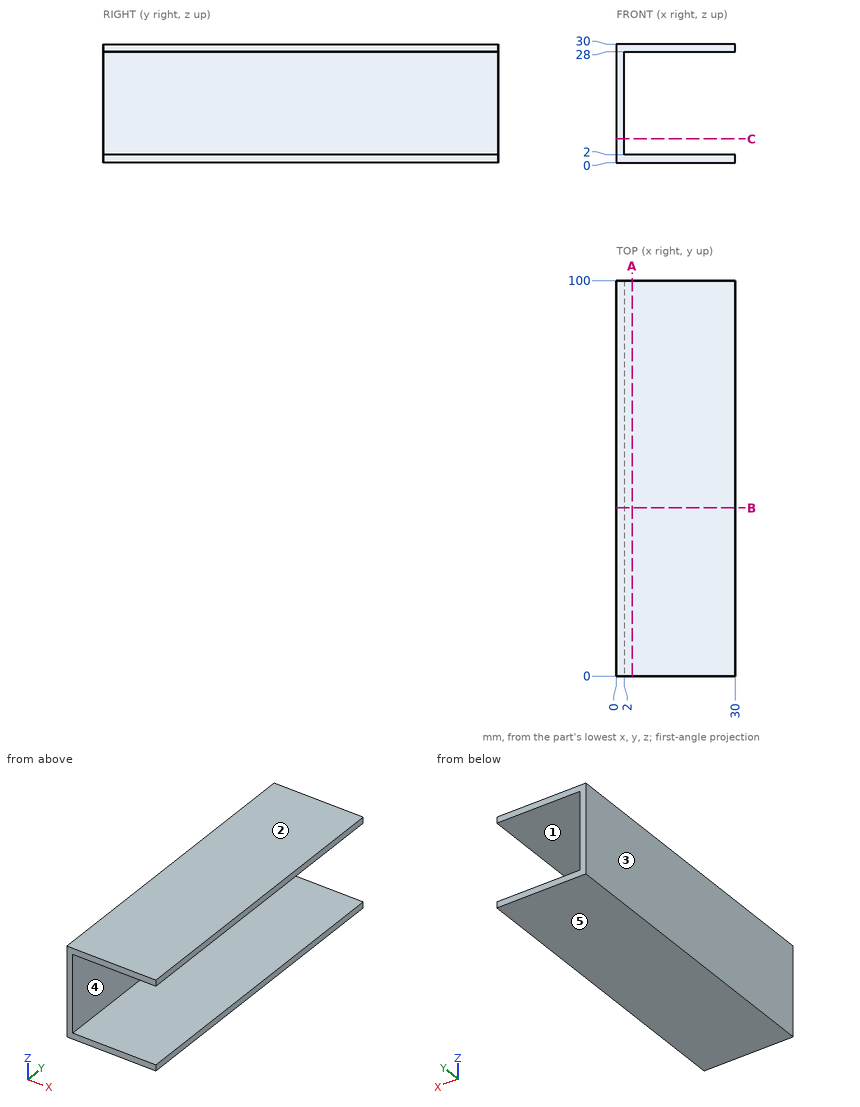
Geometry check sheet. Reference: drawing and pictorial views, mm from the part's lowest x, y, z. A direction names the side the tool comes from. Round coordinates to 2 decimals unless told otherwise and drop trailing zeros. Loops run counter-clockwise (first coordinate to the right, second up) from the corner with the lowest first, then second, coordinate; pieces in that order, holes last. Notation, with made-up numbers: (68.5, 1) - (77.5, 1) arc R23 ccw to (77.5, 28) - close; hole circle Ø8 at (-33, -22.5). An arc over 180 degrees is marked (long way). Answer in a Markdown table with one row per item. Add a question column.
Q1. Section check A-A on x = 4. Enter the section's corners in (y, z), plus the area to 3 significant figures.
Q2. Material ranges on line 1 (Z direction, x = 13.5, y = 51); line 2 (X direction, y = 25, z = 25.5), recorded low to high.
Q3. Section check C-C on z = 6. Enter the section's corners in (x, y).
Q4. Section check B-B on y = 42.5. Enter the section's corners in (x, z).
Q5. Release check for a two-part mould opening along Z. For the marked faces 3, 4 and 5 record: pulls with the +Z half, pulls with the -Z half, needs draft (parallel to the pull), parting line crosses it, or undercut.
Q6. Gauge pin test, flat end, axial feed: pin 1 (8.5 mm diameter, centred on x = 22, y = 26, fed in from -Z). Record the tip position at first contact, or that the pin passes through.
Q7. Tool access check on the marked faces 1 and 2. Record the directions out of +Z, -Z, +X, -X, +Y, -Y that give a thin tool (end or side, any length) a straight path to the whole face; none if there is none.
Found:
| question | item | result |
|---|---|---|
| 1 | outline | (0, 0) - (100, 0) - (100, 2) - (0, 2) - close; (0, 28) - (100, 28) - (100, 30) - (0, 30) - close |
| 1 | area | 400 mm² |
| 2 | line 1 | z = 0 to 2, 28 to 30 |
| 2 | line 2 | x = 0 to 2 |
| 3 | outline | (0, 0) - (2, 0) - (2, 100) - (0, 100) - close |
| 4 | outline | (0, 0) - (30, 0) - (30, 2) - (2, 2) - (2, 28) - (30, 28) - (30, 30) - (0, 30) - close |
| 5 | face 3 | needs draft |
| 5 | face 4 | undercut |
| 5 | face 5 | pulls with the -Z half |
| 6 | pin 1 | stops at z = 0 |
| 7 | face 1 | +X, +Y, -Y |
| 7 | face 2 | +Z, +X, -X, +Y, -Y |
